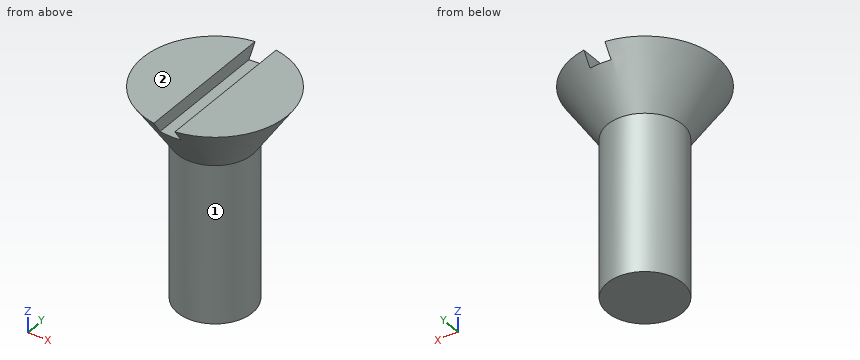
Solid Edge part; units mm, degrees
sketch "Sketch1" plane through (0, 0, 0) normal (0, 0, 1) x (1, 0, 0)
  circle A0 centre (0, 0) radius 1.425
extrude "Protrusion1" add sketch "Sketch1" against normal blind 8
sketch "Sketch2" plane through (0, 0, 0) normal (0, -1, 0) x (1, 0, 0)
  line L0 (-1.425, -2) -> (-2.75, 0)
  line L1 (-2.75, 0) -> (0, 0)
  line L2 (-1.425, -2) -> (-1.425, 0)
revolve "RevolvedProtrusion1" add sketch "Sketch2" angle 360 about axis through (0, 0, 0) along (0, 0, 1) material side at (-2.0458, 0, -0.9724)
sketch "Sketch3" plane through (0, 0, 0) normal (0, 0, 1) x (0, -1, 0)
  line L0 (-3.7678, -0.4) -> (3.7678, -0.4)
  line L1 (3.7678, -0.4) -> (3.7678, 0.4)
  line L2 (3.7678, 0.4) -> (-3.7678, 0.4)
  line L3 (-3.7678, 0.4) -> (-3.7678, -0.4)
extrude "ExtrudedCutout_1" cut sketch "Sketch3" against normal blind 0.5
properties material "Graphite"
Geometry check sheet. Reference: the model listing, model coordinates, mm. Face numbers are marked on the shaded views. A direction names the side the tool comes from. Give positions to 0.01 mm unless a question says otherwise; leave off trailing zeros. Order: outer loops, then holes, each group sorted by start corner. A loop starts at its lowest first (then second) coordinate and runs counter-clockwise, first axis right, second up.
1) Cross-section at B-B (x = 0). Record the boundary of the cut face in (y, z) (3 decimals).
Results are:
outline: (-2.419, -0.5) - (-1.425, -2) - (-1.425, -8) - (1.425, -8) - (1.425, -2) - (2.419, -0.5) - close
2) Cross-section at C-C (z = -5.75). Record the boundary of the cut face in (x, y) (3 decimals), then the cut area to 3 significant figures.
Results are:
outline: circle Ø2.85 at (0, 0)
area: 6.38 mm2
3) Cross-section at A-A (y = 0). Record the boundary of the cut face in (x, z) (3 decimals), then the cut area to 4 significant figures.
Results are:
outline: (-2.75, 0) - (-1.425, -2) - (-1.425, -8) - (1.425, -8) - (1.425, -2) - (2.75, 0) - (0.4, 0) - (0.4, -0.5) - (-0.4, -0.5) - (-0.4, 0) - close
area: 25.05 mm2
4) Material ranges on probe 1 along Z at (x, y) = (-0.65, 2.4); probe 2 along Y at (x, z) = (1.1, -4.5); probe 3 along Z at (x, y) = (1.95, -1), recorded low to high.
Results are:
probe 1: z = -0.4 to 0
probe 2: y = -0.91 to 0.91
probe 3: z = -0.84 to 0
5) Cross-section at D-D (z = -1). Record the boundary of the cut face in (x, y) (1 decimal), then the cut area to 3 significant figures.
Results are:
outline: circle Ø4.2 at (0, 0)
area: 13.7 mm2
6) Gauge pin test, flat ends, axial feed: pin 1 (0.9 mm diameter, centred on x = 0, y = -0.5, fed in from +Z); pin 2 (0.6 mm diameter, centred on y = -1, z = -0.5, fed in from -X); pin 3 (1 mm diameter, centred on y = 0.5, z = -6.5, fed in from -X) (3 decimals); pin 4 (3 mm diameter, centred on x = 2, z = -3, fed in from +Y). Record the tip position at first contact, or that the pin passes through.
Results are:
pin 1: stops at z = 0
pin 2: stops at x = -2.45
pin 3: stops at x = -1.425
pin 4: stops at y = 1.33
7) Tool access check on the marked faces 1 and 2. Record the directions out of +Z, -Z, +X, -X, +Y, -Y that give a thin tool (end or side, any length) a straight path to the whole face; none if there is none.
Results are:
face 1: -Z
face 2: +Z, +X, -X, +Y, -Y
